Can you work these out from the model? Positions are in its coordinate system, mm. A direction names the side the tool comes from. Coordinates: 2 decimals unless noted, no trailing zeros. Order: outer loops, then holes, each group sorted by start corner. A loop starts at its lowest first (then second) coordinate and runs counter-clockwise, first axis right, second up.
Autodesk Fusion 360 part; units mm, degrees
sketch "Sketch1" plane through (0, 0, 0) normal (0, 1, 0) x (1, 0, 0)
  circle A0 centre (0, 0) radius 2.75
  circle A1 centre (0, 0) radius 6.75
  dimension "d1" = 5.5
  dimension "d2" = 4
extrude "Extrude1" add sketch "Sketch1" along normal blind 12
ref_plane "WorkPlane1" through (3, 0, 0) normal (1, 0, 0) x (0, 1, 0)
sketch "Sketch2" plane through (3, 0, 0) normal (1, 0, 0) x (0, 1, 0)
  line L0 (12, -6.75) -> (12, 6.75)
  line L1 (0, -6.75) -> (0, 6.75)
  circle A0 centre (6, 0) radius 4.6
  circle A1 centre (6, 0) radius 6
  dimension "d6" = 9.2
  dimension "d7" = 6
  dimension "d8" = 12
  dimension "d9" = 1.4
extrude "Extrude2" add sketch "Sketch2" along normal blind 8
ref_plane "WorkPlane2" through (2.75, 6.403, 0) normal (-1, 0, 0) x (0, 0, -1)
sketch "Sketch3" plane through (2.75, 6.403, 0) normal (-1, 0, 0) x (0, -1, 0)
  line L0 (-5.597, -2.75) -> (-5.597, 2.75)
  line L1 (6.403, -2.75) -> (6.403, 2.75)
  line L2 (6.403, -2.75) -> (6.403, 2.75)
  line L3 (-5.597, -2.75) -> (-5.597, 2.75)
  circle A0 centre (0.403, 0) radius 3.5
  point P0 (0.403, 0)
  dimension "d13" = 6
  dimension "d14" = 12
  dimension "d20" = 7
hole "Hole1" at (2.75, 6, 0) direction (1, 0, 0) diameter 3 depth 10 tip angle 118 counterbore diameter 7 counterbore depth 2
extrude "Extrude3" cut sketch "Sketch3" along normal blind 14.5
sketch "Sketch4" plane through (0, 0, 0) normal (0, -1, 0) x (1, 0, 0)
  circle A0 centre (0, 0) radius 2.75
  circle A1 centre (0, 0) radius 6.75
  line L0 (4, 2.3094) -> (0, 4.6188)
  line L1 (0, 4.6188) -> (-4, 2.3094)
  line L2 (-4, 2.3094) -> (-4, -2.3094)
  line L3 (-4, -2.3094) -> (0, -4.6188)
  line L4 (0, -4.6188) -> (4, -2.3094)
  line L5 (4, -2.3094) -> (4, 2.3094)
  line L6 (-4.01, -2.3152) -> (0, -4.6303)
  line L7 (0, -4.6303) -> (4.01, -2.3152)
  line L8 (4.01, -2.3152) -> (4.01, 2.3152)
  line L9 (4.01, 2.3152) -> (0, 4.6303)
  line L10 (0, 4.6303) -> (-4.01, 2.3152)
  line L11 (-4.01, 2.3152) -> (-4.01, -2.3152)
  dimension "d23" = 0.01
extrude "Extrude4" cut sketch "Sketch4" against normal blind 2 contours L0 L1 L2 L3 L4 L5 | L6 L7 L8 L9 L10 L11
equation "d1 = 5 mm + 0.5 mm"
equation "d6 = 9 mm + 0.2 mm"
equation "d7 = d8 / 2"
equation "d13 = d14 / 2"
1. Imagine slicing it at B-B on x = 5.5. Please give me the cut outline in (y, z).
Completed:
outline: (0, -3.91) - (1.45, -3.91) arc R6 ccw to (10.55, -3.91) - (12, -3.91) - (12, 3.91) - (10.55, 3.91) arc R6 ccw to (1.45, 3.91) - (0, 3.91) - close; hole (3.58, -3.91) arc R4.6 ccw to (8.42, -3.91) - close; hole (3.58, 3.91) - (8.42, 3.91) arc R4.6 ccw to start; hole circle Ø3 at (6, 0)
2. I'm going to push flat-ended pins straight in: pin 1 (5 mm diameter, centred on x = -2, z = 0.5, fed in from -Y); pin 2 (5 mm diameter, centred on x = 0, z = 0, fed in from -Y); pin 3 (6.5 mm diameter, centred on y = 6, z = 0, fed in from +X); pin 4 (1.5 mm diameter, centred on x = 2, y = 5, fed in from -Z). Where does each tip first touch, or does it pass through?
Completed:
pin 1: stops at y = 0
pin 2: passes through
pin 3: stops at x = 6.75
pin 4: stops at z = -6.63
3. Imagine slicing it at D-D on y = 7. Please give me the cut outline in (x, z), then the cut area to 3 significant figures.
Completed:
outline: (-5.86, -3.35) arc R6.75 ccw to (3.25, -5.92) - (11, -5.92) - (11, -4.49) - (5.04, -4.49) arc R6.75 ccw to (6.66, -1.12) - (4.75, -1.12) - (4.75, -3.35) - close; (-5.86, 3.35) - (4.75, 3.35) - (4.75, 1.12) - (6.66, 1.12) arc R6.75 ccw to (5.04, 4.49) - (11, 4.49) - (11, 5.92) - (3.25, 5.92) arc R6.75 ccw to start
area: 82.8 mm2
4. Imagine slicing it at A-A on y = 10. Please give me the cut outline in (x, z), then the cut area to 3 significant figures.
Completed:
outline: (5.06, -4.47) - (11, -4.47) - (11, -2.27) - (6.36, -2.27) arc R6.75 ccw to (6.36, 2.27) - (11, 2.27) - (11, 4.47) - (5.06, 4.47) arc R6.75 ccw (long way) to start; hole circle Ø5.5 at (0, 0)
area: 142 mm2
5. Please list where these lines run through material, in increasing order: probe 1 along Y at (x, z) = (6.5, 0); probe 2 along Z at (x, y) = (5.25, 6); probe 3 along Z at (x, y) = (5.6, 6).
Completed:
probe 1: y = 0 to 4.5, 7.5 to 12
probe 2: z = -6 to -4.6, -4.24 to -1.5, 1.5 to 4.24, 4.6 to 6
probe 3: z = -6 to -4.6, -3.77 to -1.5, 1.5 to 3.77, 4.6 to 6
6. On a 3-axis mill with a long thin cutter (end or side, diameter ignored), from which of +Z, -Z, +X, -X, +Y, -Y can I reach the whole of each face in a straight line? I mean faces 1 (the cylindrical face through (5.764, 4.513, -0.195)), 2 (the flat face through (2.03, 0.99, 3.46)), 3 (the cylindrical face through (8.601, 8.123, 4.081)), 4 (the flat face through (4.75, 8, 0)). Say none if no direction works.
Completed:
face 1: +X, -X
face 2: -Y
face 3: +X
face 4: -X
7. Thinking about a two-plate mould opening in Z: for faces 5 (the flat face through (4.01, 1, 0)), 6 (the cylindrical face through (-5.357, 5.916, -4.107)), 7 (the flat face through (4.4, 0, -0.1)), which applies, pulls with the +Z half, pulls with the -Z half, needs draft (parallel to the pull), parting line crosses it, or undercut?
Completed:
face 5: undercut
face 6: parting line crosses it
face 7: needs draft
